from build123d import *

# Parameters (mm, degrees)
F0_W           = 152.4
F0_H           = 152.4
F1_DEPTH       = 6.35
F3_DEPTH       = 6.351
F4_R           = 2.54
F5_SIZE        = 1.27
F7_D           = 6.5278
F7_CSINK_D     = 13.4874
F7_CSINK_ANGLE = 82


with BuildPart() as f1:
    # F0 (on Top) → F1 (new body)
    with BuildSketch(Plane.XY):
        Rectangle(F0_W, F0_H)
    extrude(amount=F1_DEPTH)

    # F2 (on face) → F3 (cut, through all)
    with BuildSketch(Plane.XY.offset(6.35)):
        with BuildLine():
            Line((7.529644, 10.16), (7.529644, 38.1))
            ThreePointArc((7.529644, 38.1), (0, 45.629644), (-7.529644, 38.1))
            Line((-7.529644, 38.1), (-7.529644, 10.16))
            Line((-7.529644, 10.16), (-11.520356, 10.16))
            Line((-11.520356, 10.16), (-11.520356, 38.1))
            ThreePointArc((-11.520356, 38.1), (-19.05, 45.629644), (-26.579644, 38.1))
            Line((-26.579644, 38.1), (-26.579644, 0))
            Line((-26.579644, 0), (-26.579644, -8.89))
            Line((-26.579644, -8.89), (-45.629644, -8.89))
            Line((-45.629644, -8.89), (-45.629644, -38.1))
            ThreePointArc((-45.629644, -38.1), (-38.1, -45.629644), (-30.570356, -38.1))
            Line((-30.570356, -38.1), (-30.570356, -23.9268))
            Line((-30.570356, -23.9268), (-26.579644, -23.9268))
            Line((-26.579644, -23.9268), (-26.579644, -38.1))
            ThreePointArc((-26.579644, -38.1), (-19.05, -45.629644), (-11.520356, -38.1))
            Line((-11.520356, -38.1), (-11.520356, -10.16))
            Line((-11.520356, -10.16), (-7.529644, -10.16))
            Line((-7.529644, -10.16), (-7.529644, -38.1))
            ThreePointArc((-7.529644, -38.1), (0, -45.629644), (7.529644, -38.1))
            Line((7.529644, -38.1), (7.529644, -10.16))
            Line((7.529644, -10.16), (11.520356, -10.16))
            Line((11.520356, -10.16), (11.520356, -38.1))
            ThreePointArc((11.520356, -38.1), (19.05, -45.629644), (26.579644, -38.1))
            Line((26.579644, -38.1), (26.579644, -16.761795))
            ThreePointArc((26.579644, -16.761795), (28.227842, -11.088573), (32.659292, -7.181625))
            ThreePointArc((32.659292, -7.181625), (42.113371, 1.15348), (45.629644, 13.256762))
            Line((45.629644, 13.256762), (45.629644, 38.1))
            ThreePointArc((45.629644, 38.1), (38.1, 45.629644), (30.570356, 38.1))
            Line((30.570356, 38.1), (30.570356, 10.16))
            Line((30.570356, 10.16), (26.579644, 10.16))
            Line((26.579644, 10.16), (26.579644, 38.1))
            ThreePointArc((26.579644, 38.1), (19.05, 45.629644), (11.520356, 38.1))
            Line((11.520356, 38.1), (11.520356, 10.16))
            Line((11.520356, 10.16), (7.529644, 10.16))
        make_face()
    extrude(amount=-F3_DEPTH, mode=Mode.SUBTRACT)

    # F4
    f4_edges = [f1.edges().sort_by_distance(p)[0] for p in [
        (-7.529644, 10.16, 3.175),
        (-11.520356, -10.16, 3.175),
        (7.529644, -10.16, 3.175),
        (11.520356, 10.16, 3.175),
        (30.570356, 10.16, 3.175),
        (-26.579644, -8.89, 3.175),
        (-45.629644, -8.89, 3.175),
    ]]
    fillet(f4_edges, radius=F4_R)

    # F5
    f5_edges = [f1.edges().sort_by_distance(p)[0] for p in [
        (45.629644, 25.678381, 6.35),
        (30.570356, 25.4, 0),
        (-45.629644, -24.765, 6.35),
        (-30.570356, -31.0134, 0),
    ]]
    chamfer(f5_edges, length=F5_SIZE)

    # F7 (through all)
    with Locations(Plane.XY.offset(6.35)):
        with Locations((-63.5, 57.15), (63.5, 57.15), (63.5, -57.15), (-63.5, -57.15)):
            CounterSinkHole(F7_D / 2, F7_CSINK_D / 2, counter_sink_angle=F7_CSINK_ANGLE)


solid = f1.part
Input: part model. Units: mm. Frame: model coordinates. A direction names the side the tool comes from. Coordinates: 2 decimals unless noted, no trailing zeros. Order: outer loops, then holes, each group sorted by start corner. A loop starts at its lowest first (then second) coordinate and runs counter-clockwise, first axis right, second up. Notation, with made-up numbers: M 42,-9.75 L 57,-9.75 A30 ccw 57,18.25 Z; hole C -2.75,35 d10. An arc over 180 degrees is marked long. Answer as CSV lines item,"result".
1. Section C-C (x = -38.1). Return the cut outline in (y, z).
Reported:
outline,"M -76.2,0 L -46.9,0 L -45.63,1.27 L -45.63,5.08 L -46.9,6.35 L -76.2,6.35 Z; M -8.89,1.27 L -7.62,0 L 76.2,0 L 76.2,6.35 L -7.62,6.35 L -8.89,5.08 Z"
2. Material intervals for line 1 (Y direction, x = -63.5, z = 1.15); line 2 (X direction, y = 57.15, z = 0.75); line 3 (X direction, y = -57.5, z = 1), sorted ascending. Write a range as from..to.
Reported:
line 1,"-76.2..-60.41, -53.89..53.89, 60.41..76.2"
line 2,"-76.2..-66.76, -60.24..60.24, 66.76..76.2"
line 3,"-76.2..-66.75, -60.25..60.25, 66.75..76.2"
3. Section B-B (y = -57.15). Return the cut outline in (x, z), then the cut area to 3 significant figures.
Reported:
outline,"M -76.2,0 L -66.76,0 L -66.76,2.35 L -70.24,6.35 L -76.2,6.35 Z; M -60.24,0 L 60.24,0 L 60.24,2.35 L 56.76,6.35 L -56.76,6.35 L -60.24,2.35 Z; M 66.76,0 L 76.2,0 L 76.2,6.35 L 70.24,6.35 L 66.76,2.35 Z"
area,"857 mm2"
4. Section D-D (z = 4). State how many separate pieces and enclosed holes the cut face has, then the cut area to 3 significant figures.
Reported:
separate pieces,"1"
enclosed holes,"5"
area,"17,400 mm2"
5. First-contact query: P1, Ø8.5, axis at x = -63.5, y = -57.15, coming from the -Z side. Flat tip, straight axial feed; report the tip coordinate or a pass-through.
Reported:
P1,"z = 0"
6. Pull-direction query (X, two-part tool) for faces 4 (the conical face through (63.95, 60.55, 2.54)), 5 (the flat face through (-35, 1, 0)); classes: released by +X, released by -X, zero draft, split by the parting line, or undercut.
Reported:
face 4,"undercut"
face 5,"zero draft"
7. Section A-A (x = -19.05). Return the cut outline in (y, z).
Reported:
outline,"M -76.2,0 L -45.63,0 L -45.63,6.35 L -76.2,6.35 Z; M 45.63,1.27 L 46.9,0 L 76.2,0 L 76.2,6.35 L 46.9,6.35 L 45.63,5.08 Z"
8. Access query for faces 1 (the flat face through (26.58, 24, 3)), 2 (the conical face through (-38.27, -45.85, 5.3)), 3 (the flat face through (-35, 1, 6.35)). Directions: +Z, -Z, +X, -X, +Y, -Y. A direction counts if a zero-diameter tool reaches every point of the face in a straight line with its end or side. Return the directions, or none.
Reported:
face 1,"+Z, -Z"
face 2,"+Z"
face 3,"+Z, +X, -X, +Y, -Y"
